Read the model definition and answer for the solid it produces. Units are mm, in the model's axes. Face numbers are marked on the shaded views. A direction names the side the tool comes from. Coordinates: 2 decimals unless noted, no trailing zeros. Order: outer loops, then holes, each group sorted by start corner. A loop starts at its lowest first (then second) coordinate and runs counter-clockwise, first axis right, second up.
Autodesk Inventor part; units mm, degrees
ref_plane "YZ Plane" through (0, 0, 0) normal (1, 0, 0) x (0, 1, 0)
ref_plane "XZ Plane" through (0, 0, 0) normal (0, 1, 0) x (-1, 0, 0)
ref_plane "XY Plane" through (0, 0, 0) normal (0, 0, 1) x (1, 0, 0)
sketch "Sketch1" plane through (0, 0, 0) normal (0, 1, 0) x (-1, 0, 0)
  circle A0 centre (0, 0) radius 27.5
  dimension "d0" = 55
extrude "Extrusion1" add sketch "Sketch1" along normal blind 22
sketch "Sketch2" plane through (0, 22, 0) normal (0, 1, 0) x (1, 0, 0)
  circle A0 centre (0, 0) radius 14.5
  dimension "d3" = 29
extrude "Extrusion2" cut sketch "Sketch2" against normal blind 3.5
sketch "Sketch3" plane through (0, 0, 0) normal (0, -1, 0) x (1, 0, 0)
  circle A0 centre (0, 0) radius 14.5
extrude "Extrusion3" cut sketch "Sketch3" against normal blind 3.5
sketch "Sketch4" plane through (0, 3.5, 0) normal (0, -1, 0) x (1, 0, 0)
  circle A0 centre (0, 0) radius 7.5
  dimension "d8" = 15
extrude "Extrusion4" cut sketch "Sketch4" against normal blind 36.5
properties part number "wheel" material "EIFS, Exterior Insulation"
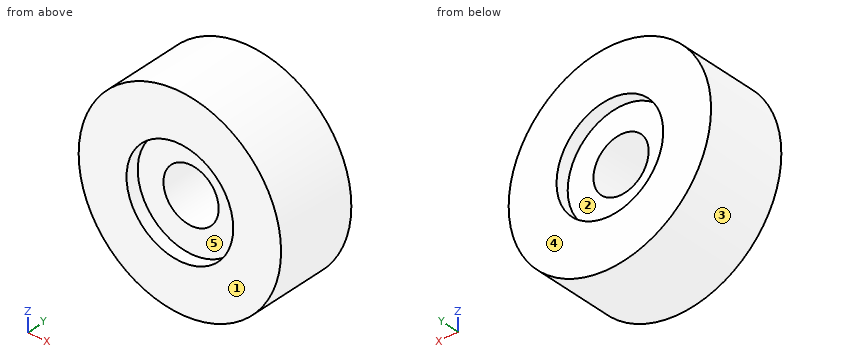
Q1. The part is cut by section B-B, the plane z = 0. Determine the outline of the cut face in (x, y).
Q2. Which of the six approach directions +Z, -Z, +X, -X, +Y, -Y give full straight-line access (tool end or side, diameter ignored) to the marked faces 4 and 5?
Q3. The part is cut by section D-D, the plane z = -13. Determine the outline of the cut face in (x, y).
Q4. Each of these flat-tipped pins is pushed along its axis until it touches: P1, Ø8.5, axis at x = -7, z = 0, coming from the +Y side; P2, Ø3, axis at y = 15, z = -7.5, coming from the +X side; P3, Ø6, axis at y = 18.5, z = 17, coming from the +X side; P4, Ø9, axis at x = 0, z = 0, coming from the +Y side. Where does it stop, or does it pass through?
Q5. The part is cut by section C-C, the plane y = 15.25. Determine the outline of the cut face in (x, z).
Q6. The part is cut by section A-A, the plane x = 0. Determine the outline of the cut face in (y, z).
Q7. Straight lines are drawn through the part: L1, parallel to Z at x = 0, y = 2.6; L2, parallel to Z at x = 0, y = 10.75; L3, parallel to Y at x = -4.5, z = -11. For each, find the intervals that lie inside material, in ascending order.
Q8. Determine the mould class of the marked faces 1, 2 and 3 for opening direction Z: +Z half, -Z half, draft (parallel to the pull), parting line (faces both ways), or undercut.
Computed values:
1. outline: (-27.5, 0) - (-14.5, 0) - (-14.5, 3.5) - (-7.5, 3.5) - (-7.5, 18.5) - (-14.5, 18.5) - (-14.5, 22) - (-27.5, 22) - close; (7.5, 3.5) - (14.5, 3.5) - (14.5, 0) - (27.5, 0) - (27.5, 22) - (14.5, 22) - (14.5, 18.5) - (7.5, 18.5) - close
2. face 4: +Z, -Z, +X, -X, +Y
2. face 5: -Y
3. outline: (-24.23, 0) - (-6.42, 0) - (-6.42, 3.5) - (6.42, 3.5) - (6.42, 0) - (24.23, 0) - (24.23, 22) - (6.42, 22) - (6.42, 18.5) - (-6.42, 18.5) - (-6.42, 22) - (-24.23, 22) - close
4. P1: stops at y = 18.5
4. P2: stops at x = 26.84
4. P3: stops at x = 23.67
4. P4: passes through
5. outline: circle Ø55 at (0, 0); hole circle Ø15 at (0, 0)
6. outline: (0, -27.5) - (22, -27.5) - (22, -14.5) - (18.5, -14.5) - (18.5, -7.5) - (3.5, -7.5) - (3.5, -14.5) - (0, -14.5) - close; (0, 14.5) - (3.5, 14.5) - (3.5, 7.5) - (18.5, 7.5) - (18.5, 14.5) - (22, 14.5) - (22, 27.5) - (0, 27.5) - close
7. L1: z = -27.5 to -14.5, 14.5 to 27.5
7. L2: z = -27.5 to -7.5, 7.5 to 27.5
7. L3: y = 3.5 to 18.5
8. face 1: draft
8. face 2: undercut
8. face 3: parting line
